The listing builds one solid part. Answer for the finished solid, in the listing's coordinates (mm). Face numbers are marked on the shaded views. A direction names the side the tool comes from. Round coordinates to 2 decimals unless told otherwise and drop trailing zeros. Order: outer loops, then holes, each group sorted by start corner. A loop starts at its lowest first (then second) coordinate and runs counter-clockwise, first axis right, second up. Notation, with made-up numbers: (64, -18.75) -> (104, -18.75) arc R37 ccw to (104, 17.25) -> close; hole circle Ø11 at (6, 3). An arc over 180 degrees is marked (long way). Answer in a Markdown table with one row per item. Add a question column.
```python
from build123d import *

# Parameters (mm, degrees)
SKETCH001_W      = 90
SKETCH001_H      = 20
SKETCH001_R      = 6
EXTRUDE001_DEPTH = 5
SKETCH_W         = 70
SKETCH_H         = 12
SKETCH_R         = 2.25
EXTRUDE_DEPTH    = 10
CHAMFER_SIZE     = 0.8


with BuildPart() as extrude001:
    # Sketch001 → Extrude001 (new body)
    with BuildSketch(Plane.XY):
        with Locations((38, 0)):
            Rectangle(SKETCH001_W, SKETCH001_H)
        with Locations((6, 0)):
            Circle(SKETCH001_R, mode=Mode.SUBTRACT)
    extrude(amount=EXTRUDE001_DEPTH)


with BuildPart() as extrude001_1:
    # Extrude001 placement: moved
    add(extrude001.part.moved(Location((0, 0, 5))))


with BuildPart() as chamfer_body:
    # Sketch → Extrude (new body)
    with BuildSketch(Plane.XY):
        with Locations((35, 0)):
            Rectangle(SKETCH_W, SKETCH_H)
        with Locations((6, 0)):
            Circle(SKETCH_R, mode=Mode.SUBTRACT)
        with BuildLine():
            ThreePointArc((20, 2.1), (17.9, 0), (20, -2.1))
            Line((20, -2.1), (65, -2.1))
            ThreePointArc((65, -2.1), (67.1, 0), (65, 2.1))
            Line((20, 2.1), (65, 2.1))
        make_face(mode=Mode.SUBTRACT)
    extrude(amount=EXTRUDE_DEPTH)

    # Cut: cut Extrude001
    add(extrude001_1.part, mode=Mode.SUBTRACT)

    # Chamfer
    chamfer_edges = [chamfer_body.edges().sort_by_distance(p)[0] for p in [
        (3.75, 0, 0),
        (3.75, 0, 10),
    ]]
    chamfer(chamfer_edges, length=CHAMFER_SIZE)


solid = chamfer_body.part
```
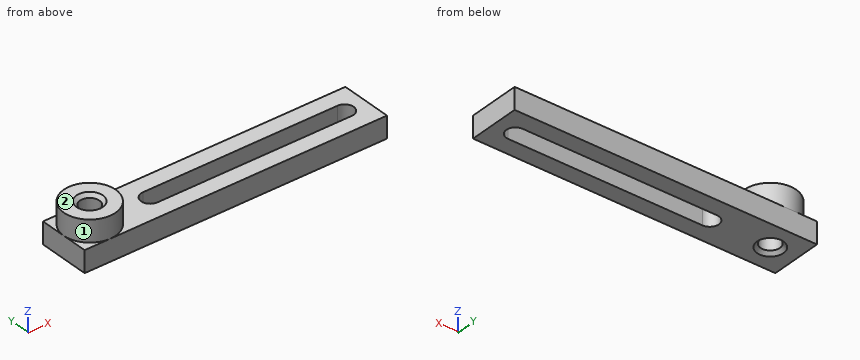
Item 1: The part is cut by section A-A, the plane x = 40.5. Give the vertices of the cut face in (y, z).
Item 2: The part is cut by section D-D, the plane x = 10.5. Give the vertices of the cut face in (y, z), and give its area (3 significant figures).
Item 3: The part is cut by section B-B, the plane z = 2.5. Give the vertices of the cut face in (x, y), and give its area (3 significant figures).
Item 4: A tool of negligible diameter and unlimited length cuts with its end or side. For the marked faces 1 and 2, from which of +Z, -Z, +X, -X, +Y, -Y can it reach the whole face along a straight path? Write none if from no direction.
Item 5: Flat-ended cylindrical pins translate along their axes: P1, Ø5, axis at x = 6, y = 0, coming from the +Z side; P2, Ø1, axis at x = 58.5, y = -2, coming from the +Z side; P3, Ø4, axis at x = 20, y = 0, coming from the -Z side. Find the tip coordinate at first contact, or state that the pin passes through.
Item 6: Find the intervals of material crossed by probe 1 along Y at (x, z) = (6, 4.5); probe 2 along Y at (x, z) = (60.5, 0.5); probe 3 along X at (y, z) = (-1.75, 3.5), in increasing order. Write a range as [from, to].
Item 7: The part is cut by section C-C, the plane y = 5. Give the vertices of the cut face in (x, z), and give its area (3 significant figures).
Resolved:
| question | item | result |
|---|---|---|
| 1 | outline | (-6, 0) -> (-2.1, 0) -> (-2.1, 5) -> (-6, 5) -> close; (2.1, 0) -> (6, 0) -> (6, 5) -> (2.1, 5) -> close |
| 2 | outline | (-6, 0) -> (6, 0) -> (6, 5) -> (3.97, 5) -> (3.97, 10) -> (-3.97, 10) -> (-3.97, 5) -> (-6, 5) -> close |
| 2 | area | 99.7 mm2 |
| 3 | outline | (0, -6) -> (70, -6) -> (70, 6) -> (0, 6) -> close; hole circle Ø4.5 at (6, 0); hole (20, -2.1) -> (65, -2.1) arc R2.1 ccw to (65, 2.1) -> (20, 2.1) arc R2.1 ccw to start |
| 3 | area | 621 mm2 |
| 4 | face 1 | +Z |
| 4 | face 2 | +Z, +X, -X, +Y, -Y |
| 5 | P1 | z = 9.45 |
| 5 | P2 | z = 5 |
| 5 | P3 | through |
| 6 | probe 1 | [-6, -2.25], [2.25, 6] |
| 6 | probe 2 | [-6, -2.1], [2.1, 6] |
| 6 | probe 3 | [0, 4.59], [7.41, 18.84], [66.16, 70] |
| 7 | outline | (0, 0) -> (70, 0) -> (70, 5) -> (9.32, 5) -> (9.32, 10) -> (2.68, 10) -> (2.68, 5) -> (0, 5) -> close |
| 7 | area | 383 mm2 |
